```python
from build123d import *

# Parameters (mm, degrees)
F0_R     = 88.94259
F1_DEPTH = 12.7
F2_SIZE  = 2.54
F3_SIZE  = 2.54
F4_R     = 53.975015
F5_DEPTH = 50.8


with BuildPart() as f1:
    # F0 (on Top) → F1 (new body)
    with BuildSketch(Plane.XY):
        Circle(F0_R)
    extrude(amount=F1_DEPTH)

    # F2
    f2_edges = [f1.edges().sort_by_distance(p)[0] for p in [
        (-88.94259, 0, 12.7),
    ]]
    chamfer(f2_edges, length=F2_SIZE)

    # F3
    f3_edges = [f1.edges().sort_by_distance(p)[0] for p in [
        (-88.94259, 0, 0),
    ]]
    chamfer(f3_edges, length=F3_SIZE)

    # F4 (on Top) → F5 (cut)
    with BuildSketch(Plane.XY):
        Circle(F4_R)
    extrude(amount=F5_DEPTH, mode=Mode.SUBTRACT)


solid = f1.part
```
For this review, take the finished solid that the model builds, in its own axes (mm). Round coordinates to 2 decimals unless told otherwise and drop trailing zeros. Order: outer loops, then holes, each group sorted by start corner. A loop starts at its lowest first (then second) coordinate and runs counter-clockwise, first axis right, second up.
Q1. We need section C-C, the plane z = 6.25. Give the boundary of the cut face in (x, y).
Findings below:
outline: circle Ø177.89 at (0, 0); hole circle Ø107.95 at (0, 0)
Q2. Wall thickness on line 1 (Y direction, x = 0, z = 7.25); line 2 (Y direction, x = -6, z = 3); line 3 (X direction, y = 23.5, z = 5.75): over which ranges is each line inside the solid? List them lowest first.
Findings below:
line 1: y = -88.94 to -53.98, 53.98 to 88.94
line 2: y = -88.74 to -53.64, 53.64 to 88.74
line 3: x = -85.78 to -48.59, 48.59 to 85.78
Q3. Insertion check: P1, Ø3, axis at x = 61, z = 8, coming from the -Y side; P2, Ø1, axis at x = -48.5, z = 5, coming from the -Y side; P3, Ø4, axis at x = 19.5, z = 11.5, coming from the -Y side. Each pin has a flat end and moves straight along its axis. Give the tip position at first contact, or say it passes through.
Findings below:
P1: stops at y = -66.11
P2: stops at y = -74.88
P3: stops at y = -87.1
Q4. Mouldability with a two-part tool opening along X and no side actions: class faces 1 (the conical face through (-18.757, -84.468, 12.577)), 2 (the cylindrical face through (51.483, 16.213, 6.261)), 3 (the flat face through (37, 40, 0)) as pulls with the +X half, pulls with the -X half, needs draft (parallel to the pull), parting line crosses it, or undercut.
Findings below:
face 1: parting line crosses it
face 2: undercut
face 3: needs draft
Q5. We need section A-A, the plane x = 0. Give the boundary of the cut face in (y, z), plus the area to 3 significant figures.
Findings below:
outline: (-88.94, 2.54) - (-86.4, 0) - (-53.98, 0) - (-53.98, 12.7) - (-86.4, 12.7) - (-88.94, 10.16) - close; (53.98, 0) - (86.4, 0) - (88.94, 2.54) - (88.94, 10.16) - (86.4, 12.7) - (53.98, 12.7) - close
area: 875 mm2
